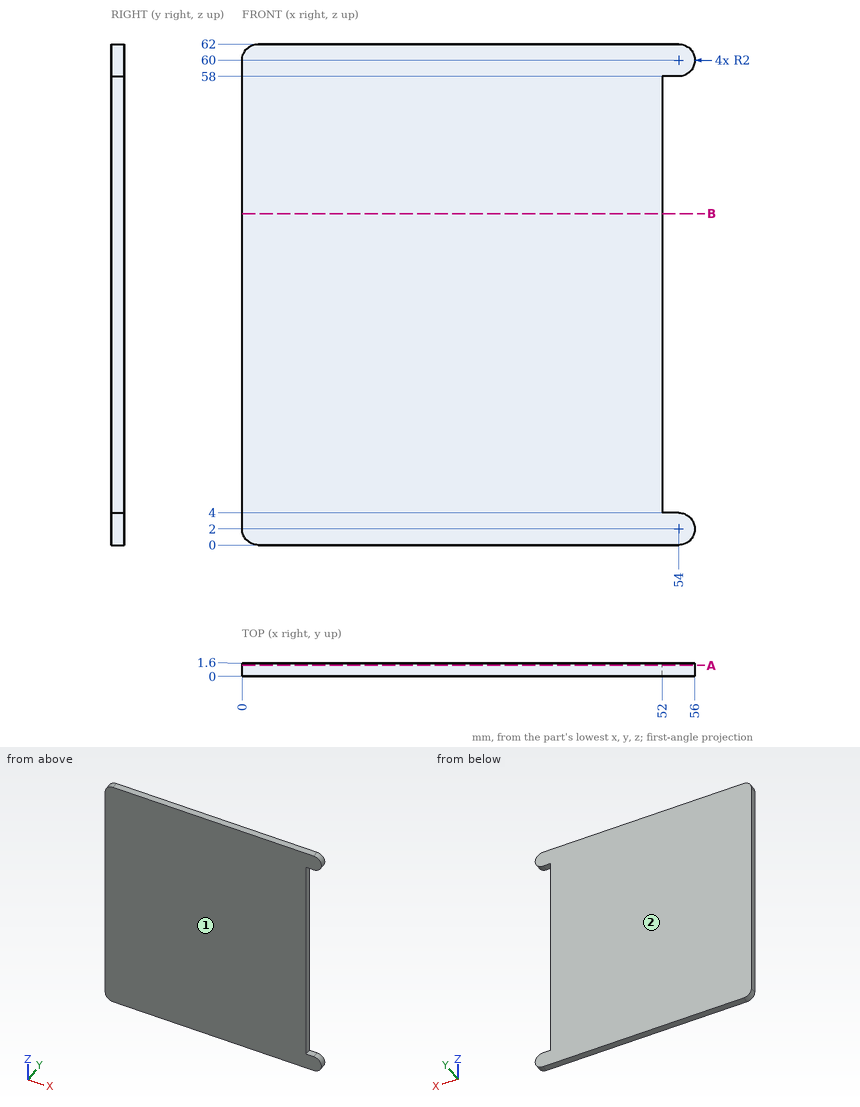
Geometry check sheet. Reference: drawing and pictorial views, mm from the part's lowest x, y, z. Coordinates: 2 decimals unless noted, no trailing zeros. Order: outer loops, then holes, each group sorted by start corner. A loop starts at its lowest first (then second) coordinate and runs counter-clockwise, first axis right, second up.
Item 1: Scan line: line 1 along X through (y, z) = (1.2, 37.5). Record every from-to range of solid material in increasing order.
Item 2: Mould release check, pull along Y, two halves, no side actions. Record for the marked faces 1 and 2: released by +Y, released by -Y, zero draft, split by the parting line, or undercut.
Item 3: Section check A-A (y = 1.3). Enter the section's corners in (x, z), plus the area to 3 significant figures.
Item 4: Section check B-B (z = 41). Enter the section's corners in (x, y), plus the area to 3 significant figures.
Item 5: Depth check by flat-ended pin: pin 1 (0.8 mm diameter, centred on y = 1, z = 25, fed in from +X). Enter the tip coordinate at first touch or a pass-through.
Check sheet entries:
1. line 1: x = 0 to 52
2. face 1: released by -Y
2. face 2: released by +Y
3. outline: (0, 2) arc R2 ccw to (2, 0) - (54, 0) arc R2 ccw to (54, 4) - (52, 4) - (52, 58) - (54, 58) arc R2 ccw to (54, 62) - (2, 62) arc R2 ccw to (0, 60) - close
3. area: 3,250 mm2
4. outline: (0, 0) - (52, 0) - (52, 1.6) - (0, 1.6) - close
4. area: 83.2 mm2
5. pin 1: stops at x = 52
